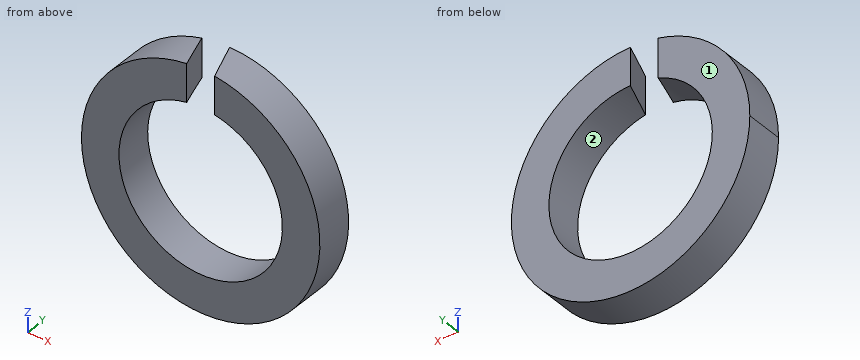
```python
from build123d import *

# Parameters (mm, degrees)
SKE_W     = 1.4
SKE_H     = 1.4
CUT_REACH = 6.45


with BuildPart() as part:
    # Ske → Base (revolve)
    with BuildSketch(Plane.XY):
        with Locations((-3.75, 0.7)):
            Rectangle(SKE_W, SKE_H)
    revolve(axis=Axis((0, 15.759672306, 0), (0, -1, 0)))

    # Ske4 → Cut (cut, up to next)
    with BuildSketch(Plane.XY, mode=Mode.PRIVATE) as cut_sk1:
        Polygon((-0.521447109, 0), (0.521447109, 0), (0.011888781, 1.4), (-1.031005436, 1.4), align=None)
    cut_tool1 = extrude(cut_sk1.sketch, amount=CUT_REACH, mode=Mode.PRIVATE) & part.part
    add(cut_tool1.solids().sort_by_distance((-0.254779, 0.7, 0))[0], mode=Mode.SUBTRACT)


solid = part.part
```
Read the model definition and answer for the solid it produces. Units are mm, in the model's axes. Face numbers are marked on the shaded views. Give positions to 0.01 mm unless a question says otherwise; leave off trailing zeros. Write each loop counter-clockwise with the first axis right and the second up, starting at its lowest first coordinate (ties: lowest second). Pieces come first, ordered by that corner, then holes. Notation, with made-up numbers: M 89,25 L 98,25 A19 cw 98,43 Z; hole C 82,60.25 d4. An arc over 180 degrees is marked long. Put each result on its own line as item: value. Start each with the question number.
1. The part is cut by section B-B, the plane z = 2.75. Give the vertices of the cut face in (x, y).
2. For a pull along Z with two mould halves and no side action, classify the marked faces 1 and 2 as released by +Z, released by -Z, zero draft, split by the parting line, or undercut.
3. The part is cut by section D-D, the plane x = 3.75. Give the vertices of the cut face in (y, z).
4. Consider line 1 along X through (y, z) = (0.35, 0); line 2 along X through (y, z) = (1.15, 2.5); line 3 along Z through (x, y) = (-2.25, 0.75). Determine where each line is inside the solid, lowest interval first.
5. The part is cut by section C-C, the plane y = 1.2. Give the vertices of the cut face in (x, z).
6. This flat-tipped pin is pushed along its axis until it touches: pin 1 Ø1.5 at (x, z) = (-3.5, 3.5) entering from -Y. Where does it stop, or does it pass through?
7. The part is cut by section A-A, the plane x = 1.25. Give the vertices of the cut face in (y, z).
Final values:
1. outline: M -3.5,0 L -1.32,0 L -1.32,1.4 L -3.5,1.4 Z; M 1.32,0 L 3.5,0 L 3.5,1.4 L 1.32,1.4 Z
2. face 1: zero draft
2. face 2: undercut
3. outline: M 0,-2.4 L 1.4,-2.4 L 1.4,2.4 L 0,2.4 Z
4. line 1: x = -4.45 to -3.05, 3.05 to 4.45
4. line 2: x = -3.68 to -1.75, 1.75 to 3.68
4. line 3: z = -3.84 to -2.06, 2.06 to 3.84
5. outline: M -0.96,2.9 L -0.96,4.35 A4.45 ccw long 0.08,4.45 L 0.08,3.05 A3.05 cw long Z
6. pin 1: stops at y = 0
7. outline: M 0,-4.27 L 1.4,-4.27 L 1.4,-2.78 L 0,-2.78 Z; M 0,2.78 L 1.4,2.78 L 1.4,4.27 L 0,4.27 Z
